Build history of the part. All positions in model axes, mm. Round coordinates to 2 decimals unless told otherwise and drop trailing zeros. Write each loop counter-clockwise with the first axis right and the second up, starting at its lowest first coordinate (ties: lowest second). Pieces come first, ordered by that corner, then holes.
from build123d import *

# Parameters (mm, degrees)
BOSS_EXTRUDE1_DEPTH   = 0.79375
F_8_CLEARANCE_HOLE1_D = 4.9149


with BuildPart() as part:
    # Sketch1 → Boss-Extrude1 (new, symmetric)
    with BuildSketch(Plane(origin=(0, 0, 0), x_dir=(0, 0, -1), z_dir=(1, 0, 0))):
        with BuildLine():
            Line((-2.187912376, 9.921624838), (19.05, 14.605))
            Line((19.05, 14.605), (19.05, -14.605))
            Line((19.05, -14.605), (-2.187912376, -9.921624838))
            ThreePointArc((-2.187912376, -9.921624838), (-10.16, 0), (-2.187912376, 9.921624838))
        make_face()
    extrude(amount=BOSS_EXTRUDE1_DEPTH, both=True)

    # #8 Clearance Hole1 (through all)
    with Locations(Plane(origin=(0.79375, 0, 0), x_dir=(0, 0, -1), z_dir=(1, 0, 0))):
        with Locations((0, 0)):
            Hole(F_8_CLEARANCE_HOLE1_D / 2)


solid = part.part
1) Wall check: L1, parallel to Y at x = -0.25, z = 0; L2, parallel to Z at x = -0.65, y = -5.5; L3, parallel to Y at x = 0.05, z = -12.5. Give the ranges that are in metal, low to high.
Results:
L1: y = -10.4 to -2.46, 2.46 to 10.4
L2: z = -19.05 to 8.54
L3: y = -13.16 to 13.16
2) Slice it at A-A (y = 0). Write the cut outline in (x, z), plus the area to 3 significant figures.
Results:
outline: (-0.79, -19.05) - (0.79, -19.05) - (0.79, -2.46) - (-0.79, -2.46) - close; (-0.79, 2.46) - (0.79, 2.46) - (0.79, 10.16) - (-0.79, 10.16) - close
area: 38.6 mm2
3) Slice it at C-C (x = -0.2). Write the cut outline in (y, z) (3 decimals), plus the area to 3 significant figures.
Results:
outline: (-14.605, -19.05) - (14.605, -19.05) - (9.922, 2.188) arc R10.16 ccw to (-9.922, 2.188) - close; hole circle Ø4.915 at (0, 0)
area: 620 mm2
4) Mould opens along Z. For faces 1 (the cylindrical face through (-0.01, -2.18, 1.13)), 2 (the flat face through (0.01, 12.23, -8.28)), 3 (the flat face through (0.794, 0, -8)) say: released by +Z, released by -Z, zero draft, split by the parting line, or undercut.
Results:
face 1: undercut
face 2: released by +Z
face 3: zero draft
5) Slice it at D-D (z = 5.5). Write the cut outline in (x, y).
Results:
outline: (-0.79, -8.54) - (0.79, -8.54) - (0.79, 8.54) - (-0.79, 8.54) - close
6) Pin check, flat tip, straight feed: pin 1 Ø2 at (y, z) = (10.5, 2.5) entering from -X. Stop position of the tip, or through.
Results:
pin 1: stops at x = -0.79
7) Slice it at B-B (z = 0). Write the cut outline in (x, y).
Results:
outline: (-0.79, -10.4) - (0.79, -10.4) - (0.79, -2.46) - (-0.79, -2.46) - close; (-0.79, 2.46) - (0.79, 2.46) - (0.79, 10.4) - (-0.79, 10.4) - close
